Autodesk Inventor part; units mm, degrees
ref_plane "YZ Plane" through (0, 0, 0) normal (1, 0, 0) x (0, 1, 0)
ref_plane "XZ Plane" through (0, 0, 0) normal (0, 1, 0) x (-1, 0, 0)
ref_plane "XY Plane" through (0, 0, 0) normal (0, 0, 1) x (1, 0, 0)
sketch "Skizze1" plane through (0, 0, 0) normal (0, 1, 0) x (-1, 0, 0)
  line L0 (0, 0) -> (306, 0)
  line L1 (306, 0) -> (306, -1.5)
  line L2 (306, -1.5) -> (0, -1.5)
  line L3 (0, -1.5) -> (0, 0)
  dimension "d0" = 306
  dimension "d1" = 1.5
extrude "Extrusion1" add sketch "Skizze1" along normal blind 160
sketch "Skizze2" plane through (-306, 0, 0) normal (0, 0, 1) x (1, 0, 0)
  line L0 (278, 20) -> (28, 20)
  line L1 (28, 20) -> (28, 140)
  line L2 (28, 140) -> (278, 140)
  line L3 (278, 140) -> (278, 20)
  line L4 (278, 20) -> (28, 140) construction
  line L5 (28, 20) -> (278, 140) construction
  line L6 (0, 0) -> (0, 160)
  line L7 (0, 160) -> (306, 160)
  point P0 (306, 0)
  point P1 (153, 80)
  dimension "d4" = 306
  dimension "d5" = 160
  dimension "d6" = 153
  dimension "d7" = 80
  dimension "d8" = 250
  dimension "d9" = 120
hole "Bohrung1" at (-28, 20, 0) at (-28, 140, 0) at (-278, 140, 0) at (-278, 20, 0) direction (0, 0, -1) diameter 4.5 depth 11.8 tip angle 118
fillet "Rundung1" radius 3 4 edges at (-306, 160, -0.75) (-306, 0, -0.75) (0, 160, -0.75) (0, 0, -0.75)
sketch "Skizze3" plane through (-303, 0, 0) normal (0, 0, 1) x (1, 0, 0)
  arc A0 (0, 160) -> (-3, 157) centre (0, 157) ccw
  arc A1 (300, 0) -> (303, 3) centre (300, 3) ccw
  line L0 (0, 157) -> (300, 3)
  arc A2 (303, 157) -> (300, 160) centre (300, 157) ccw
  arc A3 (-3, 3) -> (0, 0) centre (0, 3) ccw
  line L1 (300, 157) -> (0, 3)
  line L2 (112, 55) -> (188, 55)
  line L3 (188, 55) -> (188, 105)
  line L4 (188, 105) -> (112, 105)
  line L5 (112, 105) -> (112, 55)
  line L6 (112, 55) -> (188, 105) construction
  line L7 (188, 55) -> (112, 105) construction
  point P0 (303, 0)
  point P1 (150, 80)
  dimension "d18" = 76
  dimension "d19" = 50
extrude "Extrusion2" cut sketch "Skizze3" against normal through all
sketch "Skizze4" plane through (-303, 0, 0) normal (0, 0, 1) x (1, 0, 0)
  line L0 (112, 105) -> (188, 105)
  line L1 (188, 105) -> (188, 55)
  line L2 (112, 105) -> (188, 55)
  line L3 (112, 55) -> (188, 55)
  line L4 (188, 105) -> (112, 55)
  line L5 (101.5, 47) -> (198.5, 47)
  line L6 (198.5, 47) -> (198.5, 113)
  line L7 (198.5, 113) -> (101.5, 113)
  line L8 (101.5, 113) -> (101.5, 47)
  line L9 (101.5, 47) -> (198.5, 113) construction
  line L10 (198.5, 47) -> (101.5, 113) construction
  point P0 (303, 0)
  point P1 (150, 80)
  dimension "d22" = 97
  dimension "d23" = 66
hole "Bohrung2" at (-201.5, 113, 0) at (-104.5, 113, 0) at (-104.5, 47, 0) at (-201.5, 47, 0) direction (0, 0, -1) diameter 8 end through all
properties part number "Deckel 2,0"
Check sheet for the modelled part. Datum: model origin and axes. Units: mm. Give positions to 0.01 mm unless a question says otherwise; leave off trailing zeros. Loops run counter-clockwise (first coordinate to the right, second up) from the corner with the lowest first, then second, coordinate; pieces in that order, holes last. Notation, with made-up numbers: M 45.25,69 L 52.25,69 A27 cw 52.25,85 Z; hole C 32.25,-30 d9. An arc over 180 degrees is marked long. Return JSON: item names as keys, results as strings. Group by question number.
1. Cross-section at B-B on z = -1.2. State how many separate pieces and enclosed holes the cut face has, plus the area to 3 significant figures.
2. Thickness scan on L1, parallel to Y at x = -278, z = -0.55; L2, parallel to X at y = 47, z = -0.4; L3, parallel to X at y = 20, z = -0.8. Record the ranges inside material, lowest first.
3. Go/stop test with a flat-tipped pin: pin 1 (7 mm diameter, centred on x = -278, y = 20, fed in from -Z). Record where the tip stops, or that it passes through.
4. Cross-section at C-C on x = -120. Record the boundary of the cut face in (y, z), plus the area to 3 significant figures.
5. Mould release check, pull along Y, two halves, no side actions. Record for faces 1 (the flat face through (-155, 43, -1.5)), 2 (the cylindrical face through (-102.1, 50.2, -0.8)), 3 (the cylindrical face through (-205.466, 47.521, -0.76)): released by +Y, released by -Y, zero draft, split by the parting line, or undercut.
6. Cross-section at A-A on y = 113. Record the boundary of the cut face in (x, z).
Return value:
{
 "1": {"separate pieces": "1", "enclosed holes": "9", "area": "44,900 mm^2"},
 "2": {"L1": "0 to 17.75, 22.25 to 137.75, 142.25 to 160", "L2": "-306 to -205.5, -197.5 to -108.5, -100.5 to 0", "L3": "-306 to -280.25, -275.75 to -30.25, -25.75 to 0"},
 "3": {"pin 1": "z = -1.5"},
 "4": {"outline": "M 0,-1.5 L 55,-1.5 L 55,0 L 0,0 Z; M 105,-1.5 L 160,-1.5 L 160,0 L 105,0 Z", "area": "165 mm^2"},
 "5": {"face 1": "zero draft", "face 2": "undercut", "face 3": "undercut"},
 "6": {"outline": "M -306,-1.5 L -205.5,-1.5 L -205.5,0 L -306,0 Z; M -197.5,-1.5 L -108.5,-1.5 L -108.5,0 L -197.5,0 Z; M -100.5,-1.5 L 0,-1.5 L 0,0 L -100.5,0 Z"}
}
